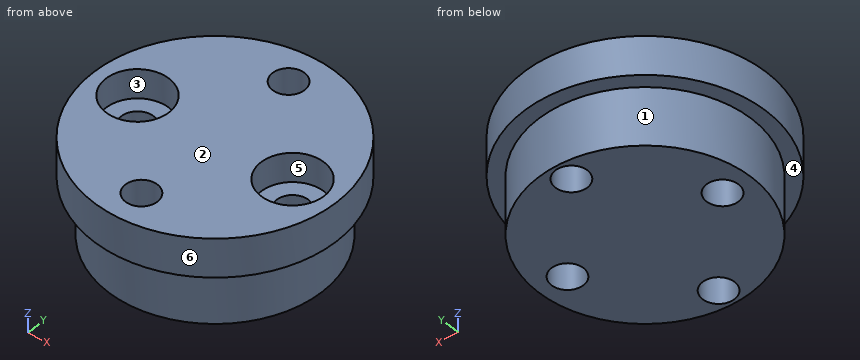
```python
from build123d import *

# Parameters (mm, degrees)
F3_D           = 3.3
F3_DEPTH       = 10
F3_TIP         = 0.9914200214
F4_D           = 3.3
F4_DEPTH       = 10
F4_CBORE_D     = 6.5
F4_CBORE_DEPTH = 3
F4_TIP         = 0.9914200214


with BuildPart() as f1:
    # F0 (on Front) → F1 (revolve)
    with BuildSketch(Plane.XZ):
        Polygon((0, 10), (0, 0), (11, 0), (11, 6), (12.5, 6), (12.5, 10), align=None)
    revolve(axis=Axis((0, 0, 5), (0, 0, -1)))

    # F3
    with Locations(Plane.XY.offset(10)):
        with Locations((0, 9), (0, -9)):
            Hole(F3_D / 2, depth=F3_DEPTH)
            with Locations((0, 0, -(F3_DEPTH + F3_TIP / 2))):  # 118° drill point
                Cone(0, F3_D / 2, F3_TIP, mode=Mode.SUBTRACT)

    # F4
    with Locations(Plane.XY.offset(10)):
        with Locations((-8, 0), (8, 0)):
            CounterBoreHole(F4_D / 2, F4_CBORE_D / 2, F4_CBORE_DEPTH, depth=F4_DEPTH)
            with Locations((0, 0, -(F4_DEPTH + F4_TIP / 2))):  # 118° drill point
                Cone(0, F4_D / 2, F4_TIP, mode=Mode.SUBTRACT)


solid = f1.part
```
Design review of the part built by this model. Coordinates are the model's own, in mm. Face numbers are marked on the shaded views. A direction names the side the tool comes from. Coordinates: 2 decimals unless noted, no trailing zeros. Write each loop counter-clockwise with the first axis right and the second up, starting at its lowest first coordinate (ties: lowest second). Pieces come first, ordered by that corner, then holes.
1) Add section D-D (x = -8.5). Write out the cut boundary in (y, z).
2) Machinability: for the marked faces 1, 2 and 3, which of the approach directions +Z, -Z, +X, -X, +Y, -Y give a long, thin tool a straight path to every point of the face, cutting with its end or side? Answer none if there is none.
3) Insertion check: pin 1 (10.5 mm diameter, centred on x = 8, y = 0, fed in from -Z); pin 2 (3 mm diameter, centred on x = -8, y = 0, fed in from -Z); pin 3 (4 mm diameter, centred on x = -8, y = 0, fed in from +Z). Each pin has a flat end and moves straight along its axis. Give the tip position at first contact, or say it passes through.
4) Add section A-A (x = 0). Write out the cut boundary in (y, z), plus the area to 3 significant figures.
5) To check wall thickness, follow L1, parallel to X at y = 0, z = 3.75; L2, parallel to Y at x = 0, z = 7.25; L3, parallel to X at y = 1, z = 2.5. State the ranges of each line that lie inside material, in increasing order.
6) Add section C-C (z = 7.5). Write out the cut boundary in (x, y).
7) Add section B-B (y = 0). Write out the cut boundary in (x, z).
8) Mouldability with a two-part tool opening along Y and no side actions: class the marked faces 4, 5 and 6 as +Y half, -Y half, draft (parallel to the pull), parting line (faces both ways), or undercut.
Check result:
1. outline: (-9.17, 6) - (-6.98, 6) - (-6.98, 0) - (-1.57, 0) - (-1.57, 7) - (-3.21, 7) - (-3.21, 10) - (-9.17, 10) - close; (1.57, 0) - (6.98, 0) - (6.98, 6) - (9.17, 6) - (9.17, 10) - (3.21, 10) - (3.21, 7) - (1.57, 7) - close
2. face 1: -Z
2. face 2: +Z, +X, -X, +Y, -Y
2. face 3: +Z
3. pin 1: stops at z = 0
3. pin 2: passes through
3. pin 3: stops at z = 7
4. outline: (-12.5, 6) - (-11, 6) - (-11, 0) - (-10.65, 0) - (-10.65, 10) - (-12.5, 10) - close; (-7.35, 0) - (7.35, 0) - (7.35, 10) - (-7.35, 10) - close; (10.65, 0) - (11, 0) - (11, 6) - (12.5, 6) - (12.5, 10) - (10.65, 10) - close
4. area: 166 mm2
5. L1: x = -11 to -9.65, -6.35 to 6.35, 9.65 to 11
5. L2: y = -12.5 to -10.65, -7.35 to 7.35, 10.65 to 12.5
5. L3: x = -10.95 to -9.31, -6.69 to 6.69, 9.31 to 10.95
6. outline: circle Ø25 at (0, 0); hole circle Ø6.5 at (-8, 0); hole circle Ø3.3 at (0, -9); hole circle Ø3.3 at (0, 9); hole circle Ø6.5 at (8, 0)
7. outline: (-12.5, 6) - (-11, 6) - (-11, 0) - (-9.65, 0) - (-9.65, 7) - (-11.25, 7) - (-11.25, 10) - (-12.5, 10) - close; (-6.35, 0) - (6.35, 0) - (6.35, 7) - (4.75, 7) - (4.75, 10) - (-4.75, 10) - (-4.75, 7) - (-6.35, 7) - close; (9.65, 0) - (11, 0) - (11, 6) - (12.5, 6) - (12.5, 10) - (11.25, 10) - (11.25, 7) - (9.65, 7) - close
8. face 4: draft
8. face 5: undercut
8. face 6: parting line
